Source: three-view drawing plus pictorial views. Frame: mm from the lowest corner of the part. Give positions to 0.01 mm unless a question says otherwise; leave off trailing zeros. Loops run counter-clockwise (first coordinate to the right, second up) from the corner with the lowest first, then second, coordinate; pieces in that order, holes last. Notation, with made-up numbers: (87.5, -1) - (133.5, -1) arc R30 ccw to (133.5, 28) - close; hole circle Ø1 at (44, 40). An arc over 180 degrees is marked (long way). Answer in a Markdown table with one row per item.
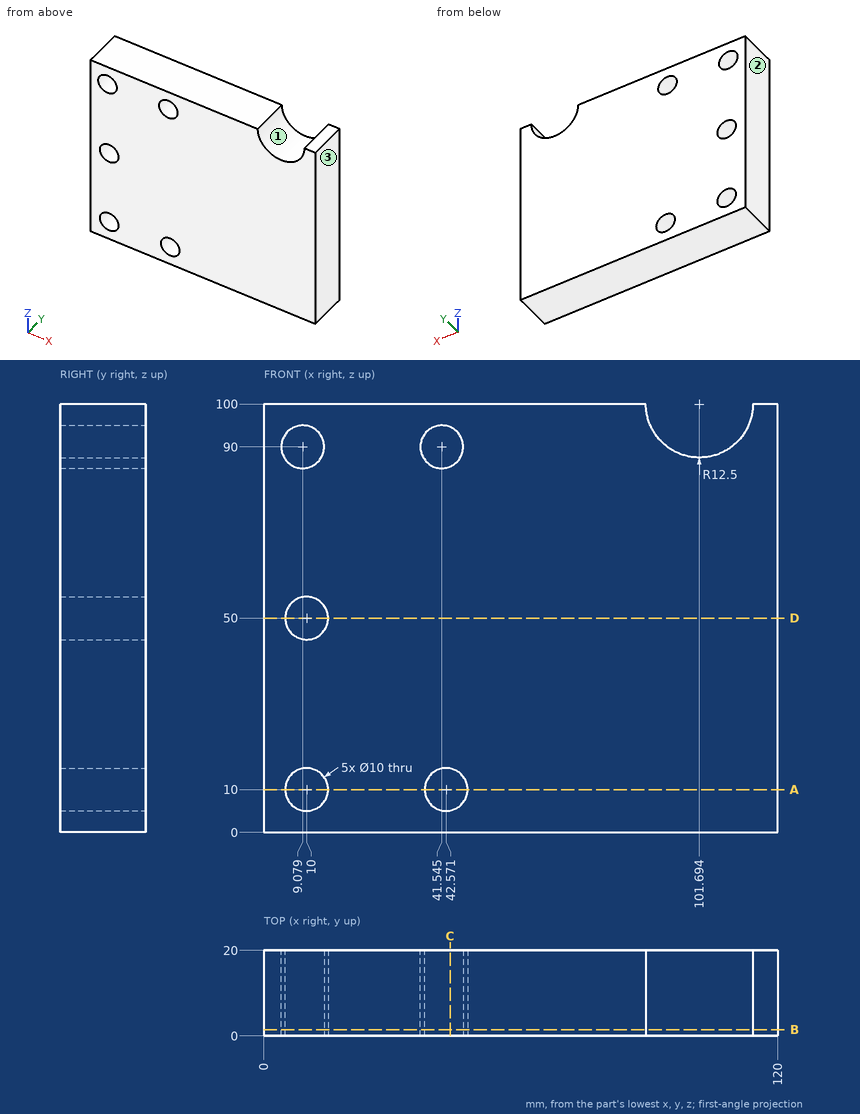
Q1. Cut plane B-B (y = 1.5). Output: boundary loops of the cut face in (x, z) (1 decimal), and give its area (3 significant figures).
Check values:
| item | result |
|---|---|
| outline | (0, 0) - (120, 0) - (120, 100) - (114.2, 100) arc R12.5 cw to (89.2, 100) - (0, 100) - close; hole circle Ø10 at (9.1, 90); hole circle Ø10 at (10, 10); hole circle Ø10 at (10, 50); hole circle Ø10 at (41.5, 90); hole circle Ø10 at (42.6, 10) |
| area | 11,400 mm² |
Q2. Cut plane C-C (x = 43.5). Output: boundary loops of the cut face in (y, z), and give its area (3 significant figures).
Check values:
| item | result |
|---|---|
| outline | (0, 0) - (20, 0) - (20, 5.09) - (0, 5.09) - close; (0, 14.91) - (20, 14.91) - (20, 85.4) - (0, 85.4) - close; (0, 94.6) - (20, 94.6) - (20, 100) - (0, 100) - close |
| area | 1,620 mm² |
Q3. Material intervals for line 1 along Z through (x, y) = (5.5, 12) (1 decimal); line 2 along X through (y, z) = (8.5, 13); line 3 along Z through (x, y) = (6, 2), sorted ascending.
Check values:
| item | result |
|---|---|
| line 1 | 0 to 7.8, 12.2 to 47.8, 52.2 to 86.5, 93.5 to 100 |
| line 2 | 0 to 6, 14 to 38.57, 46.57 to 120 |
| line 3 | 0 to 7, 13 to 47, 53 to 86.06, 93.94 to 100 |
Q4. Cut plane A-A (z = 10). Output: boundary loops of the cut face in (x, y).
Check values:
| item | result |
|---|---|
| outline | (0, 0) - (5, 0) - (5, 20) - (0, 20) - close; (15, 0) - (37.57, 0) - (37.57, 20) - (15, 20) - close; (47.57, 0) - (120, 0) - (120, 20) - (47.57, 20) - close |
Q5. Draft query along X for the marked faces 1, 2 and 3. Return one class per face: pulls with the +X half, pulls with the -X half, needs draft (parallel to the pull), parting line crosses it, or undercut.
Check values:
| item | result |
|---|---|
| face 1 | undercut |
| face 2 | pulls with the -X half |
| face 3 | pulls with the +X half |
Q6. First-contact query: pin 1 (9 mm diameter, centred on x = 10, z = 50, fed in from -Y); pin 2 (3 mm diameter, centred on x = 94.5, y = 14.5, fed in from +Z). Flat tips, straight axial feed; report the tip coordinate or a pass-through.
Check values:
| item | result |
|---|---|
| pin 1 | through |
| pin 2 | z = 91.02 |
Q7. Cut plane D-D (z = 50). Output: boundary loops of the cut face in (x, y).
Check values:
| item | result |
|---|---|
| outline | (0, 0) - (5, 0) - (5, 20) - (0, 20) - close; (15, 0) - (120, 0) - (120, 20) - (15, 20) - close |
